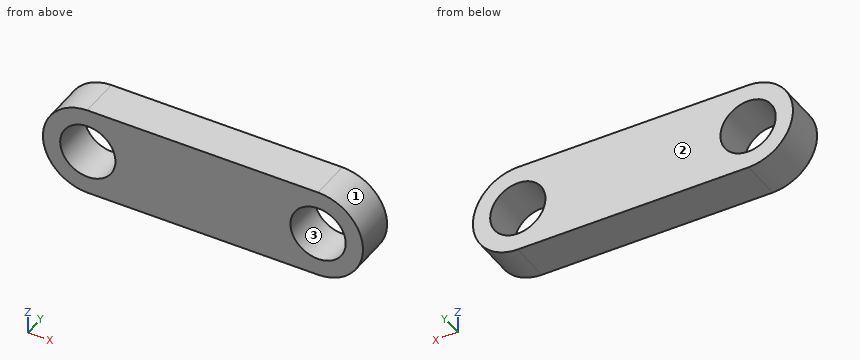
from build123d import *

# Parameters (mm, degrees)
ESQUISSE1_R             = 2.032
BOSS_EXTRU_1_DEPTH      = 3.048
ECHELLE1_SCALE          = 1.5
ESQUISSE2_R             = 3.048
ENL_V_MAT_EXTRU_1_DEPTH = 49.114943513
ESQUISSE3_R             = 3.048
ENL_V_MAT_EXTRU_2_DEPTH = 49.114943513


with BuildPart() as part:
    # Esquisse1 → Boss.-Extru.1 (new body)
    with BuildSketch(Plane(origin=(0, 0, 0), x_dir=(1, 0, 0), z_dir=(0, 1, 0))):
        with BuildLine():
            Line((0, 0), (33.782, 0))
            ThreePointArc((33.782, 0), (37.084, 3.302), (33.782, 6.604))
            Line((33.782, 6.604), (0, 6.604))
            ThreePointArc((0, 6.604), (-3.302, 3.302), (0, 0))
        make_face()
        with Locations(Location((0, 3.302, 0), (0, 0, 90))):
            Circle(ESQUISSE1_R, mode=Mode.SUBTRACT)
        with Locations(Location((33.782, 3.302, 0), (0, 0, 90))):
            Circle(ESQUISSE1_R, mode=Mode.SUBTRACT)
    extrude(amount=BOSS_EXTRU_1_DEPTH)


with BuildPart() as part_1:
    # Echelle1: scaled about (16.891, 1.524, -3.302)
    add(part.part.scale(ECHELLE1_SCALE).moved(Location((-8.4455, -0.762, 1.651))))

    # Esquisse2 → Enlèv. mat.-Extru.1 (cut, through all)
    with BuildSketch(Plane(origin=(0, 3.81, 0), x_dir=(1, 0, 0), z_dir=(0, 1, 0))):
        with Locations(Location((16.8275, 3.302, 0), (0, 0, 270))):
            Circle(ESQUISSE2_R)
    extrude(amount=-ENL_V_MAT_EXTRU_1_DEPTH, mode=Mode.SUBTRACT)

    # Esquisse3 → Enlèv. mat.-Extru.2 (cut, through all)
    # profile 1 of 3: a face of its own
    with BuildSketch(Plane(origin=(0, 3.81, 0), x_dir=(1, 0, 0), z_dir=(0, 1, 0))):
        with BuildLine():
            ThreePointArc((-13.3985, 3.301999981), (-11.947799894, 6.804299881), (-8.4455, 8.255))
            Line((-8.4455, 8.255), (-13.3985, 8.255))
            Line((-13.3985, 8.255), (-13.3985, 3.301999981))
        make_face()
    # profile 2 of 3: a face of its own
    with BuildSketch(Plane(origin=(0, 3.81, 0), x_dir=(1, 0, 0), z_dir=(0, 1, 0))):
        with BuildLine():
            ThreePointArc((-8.4455, -1.651), (-11.947799881, -0.200299894), (-13.3985, 3.301999981))
            Line((-13.3985, 3.301999981), (-13.3985, -1.651))
            Line((-13.3985, -1.651), (-8.4455, -1.651))
        make_face()
    # profile 3 of 3: a face of its own
    with BuildSketch(Plane(origin=(0, 3.81, 0), x_dir=(1, 0, 0), z_dir=(0, 1, 0))):
        with BuildLine():
            Line((16.764, 8.255), (-8.4455, 8.255))
            ThreePointArc((-8.4455, 8.255), (-11.947799894, 6.804299881), (-13.3985, 3.301999981))
            ThreePointArc((-13.3985, 3.301999981), (-11.947799881, -0.200299894), (-8.4455, -1.651))
            Line((-8.4455, -1.651), (16.764, -1.651))
            ThreePointArc((16.764, -1.651), (11.874092965, 3.302), (16.764, 8.255))
        make_face()
        with Locations((-8.4455, 3.302)):
            Circle(ESQUISSE3_R, mode=Mode.SUBTRACT)
    extrude(amount=-ENL_V_MAT_EXTRU_2_DEPTH, mode=Mode.SUBTRACT)


solid = part_1.part
Here's how the part is built. I have some questions about the finished solid (model axes, mm). Face numbers are marked on the shaded views. Round coordinates to 2 decimals unless told otherwise and drop trailing zeros. Loops run counter-clockwise (first coordinate to the right, second up) from the corner with the lowest first, then second, coordinate; pieces in that order, holes last. Notation, with made-up numbers: M 81,32 L 115,32 A29 ccw 115,53 Z; hole C 73.25,-33.75 d2. An arc over 180 degrees is marked long. Write each question's results on one line, items separated by ' | '. Start each with the question number.
(1) Thinking about a two-plate mould opening in Z: for the marked faces 1, 2 and 3, which applies, pulls with the +Z half, pulls with the -Z half, needs draft (parallel to the pull), parting line crosses it, or undercut?
(2) If I drill on probe 1 along X at (y, z) = (3, -2.5); probe 2 along X at (y, z) = (3.4, -0.75); probe 3 along Z at (x, y) = (15, 1.75), over which ranges is the centre line in solid material (lowest first)? Write a range as from..to.
(3) I want a section at D-D (x = 16). Please give me the cut outline in (y, z).
(4) I want a section at C-C (y = 2.15). State how many separate pieces and enclosed holes the cut face has, then the cut area to 3 significant figures.
(5) I want a section at A-A (x = 43). Please give me the cut outline in (y, z).
(6) I want a section at B-B (z = -1). Please give me the cut outline in (x, y), then the cut area to 3 significant figures.
(7) Will these pins go through, and if not, where does the flat tip stop? P1, Ø3.5, axis at x = 16.83, z = -3.3, coming from the +Y side; P2, Ø1, axis at x = 43, y = 1.5, coming from the -Z side; P3, Ø1.5, axis at y = 0, z = -7, coming from the -X side.
Solved:
1) face 1: parting line crosses it | face 2: needs draft | face 3: undercut
2) probe 1: x = 11.94..13.89, 19.77..39.29, 45.17..47.12 | probe 2: x = 12.58..15.16, 18.49..40.56, 43.89..46.47 | probe 3: z = -7.91..-5.74, -0.86..1.3
3) outline: M -0.76,-8.19 L 3.81,-8.19 L 3.81,-6.24 L -0.76,-6.24 Z; M -0.76,-0.37 L 3.81,-0.37 L 3.81,1.58 L -0.76,1.58 Z
4) separate pieces: 1 | enclosed holes: 2 | area: 270 mm²
5) outline: M -0.76,-8.19 L 3.81,-8.19 L 3.81,-6.25 L -0.76,-6.25 Z; M -0.76,-0.35 L 3.81,-0.35 L 3.81,1.59 L -0.76,1.59 Z
6) outline: M 12.44,-0.76 L 14.83,-0.76 L 14.83,3.81 L 12.44,3.81 Z; M 18.83,-0.76 L 40.23,-0.76 L 40.23,3.81 L 18.83,3.81 Z; M 44.23,-0.76 L 46.61,-0.76 L 46.61,3.81 L 44.23,3.81 Z | area: 120 mm²
7) P1: passes through | P2: stops at z = -8.25 | P3: stops at x = 12.85
